```python
from build123d import *

# Parameters (mm, degrees)
BOSS_EXTRUDE1_DEPTH = 6.35
BOSS_EXTRUDE2_DEPTH = 6.35
SKETCH4_W           = 12.419699812
SKETCH4_H           = 3.102298877
CUT_EXTRUDE1_DEPTH  = 7.35


with BuildPart() as part:
    # Sketch1 → Boss-Extrude1 (new body)
    with BuildSketch(Plane.XY):
        Polygon((-38.1, -20.066), (-12.7, -20.066), (-12.7, -26.416), (12.7, -26.416), (12.7, -20.066), (38.1, -20.066), (38.1, -12.7), (-38.1, 25.4), align=None)
    extrude(amount=BOSS_EXTRUDE1_DEPTH)

    # Sketch2 → Boss-Extrude2 (add, through all)
    with BuildSketch(Plane.XY.offset(6.35)):
        Polygon((38.1, -20.066), (72.644, -20.066), (72.644, -12.7), (72.644, -8.944268717), (30.588537433, -8.944268717), (38.1, -12.7), align=None)
    extrude(amount=-BOSS_EXTRUDE2_DEPTH)

    # Sketch4 → Cut-Extrude1 (cut, through all)
    with BuildSketch(Plane(origin=(0, 0, 0), x_dir=(-1, 0, 0), z_dir=(0, 0, -1))):
        with Locations((-61.565974267, -15.172394908)):
            Rectangle(SKETCH4_W, SKETCH4_H)
    extrude(amount=-CUT_EXTRUDE1_DEPTH, mode=Mode.SUBTRACT)


solid = part.part
```
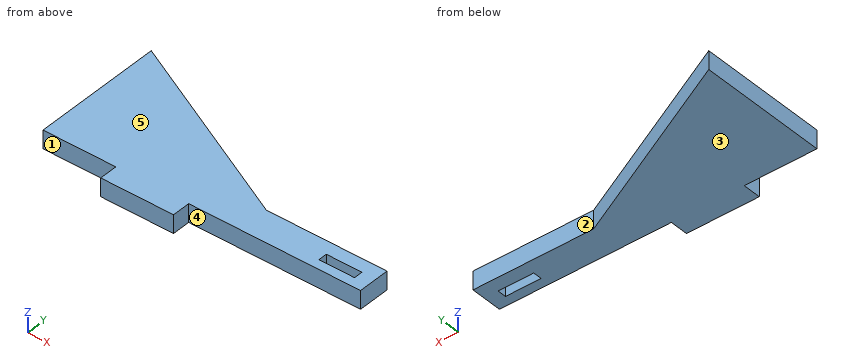
Model file for the job. Use its own axes, mm. Face numbers are marked on the shaded views. A direction names the side the tool comes from. Coordinates: 2 decimals unless noted, no trailing zeros. Order: outer loops, then holes, each group sorted by start corner. A loop starts at its lowest first (then second) coordinate and runs counter-clockwise, first axis right, second up. Notation, with made-up numbers: (28.5, 60.5) - (58.5, 60.5) arc R31 ccw to (58.5, 89.5) - close; hole circle Ø2 at (1, 85). An arc over 180 degrees is marked (long way). Return JSON: item names as keys, results as strings. Group by question number.
1) Tool access for the marked faces 1, 2, 3, 4 and 5: list every direction of +Z, -Z, +X, -X, +Y, -Y with a clear straight run to the whole face (end or side of a thin tool).
2) Flat gauge pins, fed straight in: P1, Ø3, axis at x = 62.5, z = 2, coming from the +Y side; P2, Ø1, axis at x = 27, z = 0.5, coming from the +Y side; P3, Ø1, axis at y = 14.5, z = 4, coming from the +X side. Where does each tip first touch, or does it go through?
3) Saw through at D-D, the plane x = -26. Write the cut outline in (y, z), plus the area to 3 significant figures.
4) Saw through at C-C, the plane y = -22. Write the cut outline in (x, z), plus the area to 3 significant figures.
5) Saw through at A-A, the plane x = 60. Write the cut outline in (y, z), plus the area to 3 significant figures.
6) Probe line 1 (Y direction, x = 64, z = 1.25); line 2 (X direction, y = -15.5, z = 4); line 3 (Y direction, x = 54, z = 4). List the from-to ranges inside material, lowest first. Write a range as from..to.
7) Saw through at B-B, the plane z = 2.5. Write the cut outline in (x, y), plus the area to 3 significant figures.
Values found:
{
 "1": {"face 1": "+Z, -Z, -X, -Y", "face 2": "+Z, -Z, +X, +Y", "face 3": "-Z, +X, -X, +Y, -Y", "face 4": "+Z, -Z, +X, -Y", "face 5": "+Z, +X, -X, +Y, -Y"},
 "2": {"P1": "stops at y = -8.94", "P2": "stops at y = -6.9", "P3": "stops at x = -15.3"},
 "3": {"outline": "(-20.07, 0) - (19.35, 0) - (19.35, 6.35) - (-20.07, 6.35) - close", "area": "250 mm²"},
 "4": {"outline": "(-12.7, 0) - (12.7, 0) - (12.7, 6.35) - (-12.7, 6.35) - close", "area": "161 mm²"},
 "5": {"outline": "(-20.07, 0) - (-16.72, 0) - (-16.72, 6.35) - (-20.07, 6.35) - close; (-13.62, 0) - (-8.94, 0) - (-8.94, 6.35) - (-13.62, 6.35) - close", "area": "50.9 mm²"},
 "6": {"line 1": "y = -20.07..-16.72, -13.62..-8.94", "line 2": "x = -38.1..55.36, 67.78..72.64", "line 3": "y = -20.07..-8.94"},
 "7": {"outline": "(-38.1, -20.07) - (-12.7, -20.07) - (-12.7, -26.42) - (12.7, -26.42) - (12.7, -20.07) - (72.64, -20.07) - (72.64, -8.94) - (30.59, -8.94) - (-38.1, 25.4) - close; hole (55.36, -16.72) - (67.78, -16.72) - (67.78, -13.62) - (55.36, -13.62) - close", "area": "2,530 mm²"}
}
